Can you work these out from the model? Positions are in its coordinate system, mm. Face numbers are marked on the shaded views. A direction names the side the tool comes from. Give positions to 0.01 mm unless a question says otherwise; leave off trailing zeros. Write each loop counter-clockwise with the first axis right and the second up, starting at its lowest first coordinate (ties: lowest second). Pieces come first, ordered by that corner, then holes. Notation, with made-up numbers: (61, -31.75) - (119, -31.75) arc R18 cw to (119, -13.75) - close; hole circle Ø11 at (50, 65.5). An arc over 180 degrees is marked (long way). Use a Markdown table: item, result. Add a question column.
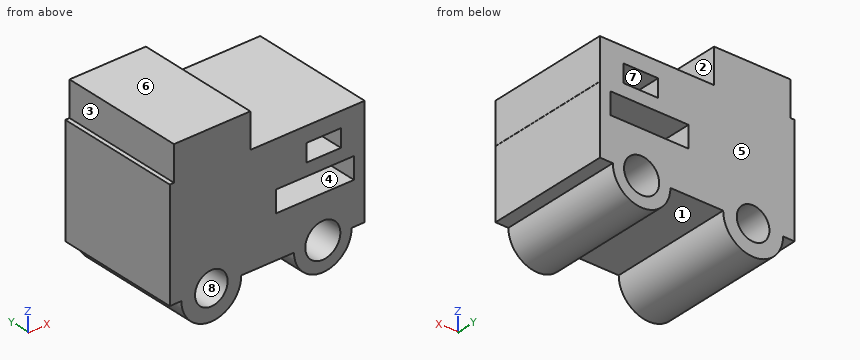
```python
from build123d import *

# Parameters (mm, degrees)
F0_W     = 21.6928645968
F0_H     = 12.4372411519
F0_W_2   = 24.2960043252
F0_W_3   = 53.6649217829
F0_H_2   = 15.3809413314
F0_W_4   = 54.884574376
F0_H_3   = 15.0760281831
F1_DEPTH = 25.4
F2_DEPTH = 62.738
F3_DEPTH = 71.374


with BuildPart() as f1:
    # F0 (on Front) → F1 (new body)
    with BuildSketch(Plane.XZ):
        Polygon((-61.0292442143, 47.0119267702), (-61.0292442143, 18.3321516961), (75.8868977427, 18.3321516961), (75.9811550379, 18.3321516961), (75.9811550379, 47.0119267702), align=None)
        with Locations((-32.8727662563, 29.9694752321)):
            Rectangle(F0_W, F0_H, mode=Mode.SUBTRACT)
        with Locations((47.1015777439, 29.9694752321)):
            Rectangle(F0_W_2, F0_H, mode=Mode.SUBTRACT)
        with BuildLine():
            Line((75.8868977427, 18.3321516961), (-61.0292442143, 18.3321516961))
            Line((-61.0292442143, 18.3321516961), (-61.0292442143, -29.6469051391))
            Line((-61.0292442143, -29.6469051391), (-52.8746465882, -29.6469051391))
            ThreePointArc((-52.8746465882, -29.6469051391), (-31.816188246, -8.5884467969), (-10.7577299038, -29.6469051391))
            Line((-10.7577299038, -29.6469051391), (26.3103456442, -29.6469051391))
            ThreePointArc((26.3103456442, -29.6469051391), (46.5673431754, -9.3899076079), (66.8243407066, -29.6469051391))
            Line((66.8243407066, -29.6469051391), (75.8868977427, -29.6469051391))
            Line((75.8868977427, -29.6469051391), (75.8868977427, 18.3321516961))
        make_face()
        with Locations((-31.2481601723, 7.6904706657)):
            Rectangle(F0_W_3, F0_H_2, mode=Mode.SUBTRACT)
        with Locations((41.0165307112, 7.5380140916)):
            Rectangle(F0_W_4, F0_H_3, mode=Mode.SUBTRACT)
        with BuildLine():
            ThreePointArc((-10.7577299038, -29.6469051391), (-31.816188246, -8.5884467969), (-52.8746465882, -29.6469051391))
            Line((-52.8746465882, -29.6469051391), (-43.2868667506, -29.6469051391))
            ThreePointArc((-43.2868667506, -29.6469051391), (-31.816188246, -18.1762266345), (-20.3455097415, -29.6469051391))
            Line((-20.3455097415, -29.6469051391), (-10.7577299038, -29.6469051391))
        make_face()
        with BuildLine():
            Line((-43.2868667506, -29.6469051391), (-52.8746465882, -29.6469051391))
            ThreePointArc((-52.8746465882, -29.6469051391), (-31.816188246, -50.7053634813), (-10.7577299038, -29.6469051391))
            Line((-10.7577299038, -29.6469051391), (-20.3455097415, -29.6469051391))
            ThreePointArc((-20.3455097415, -29.6469051391), (-31.816188246, -41.1175836436), (-43.2868667506, -29.6469051391))
        make_face()
        with BuildLine():
            ThreePointArc((26.3103456442, -29.6469051391), (46.5673431754, -49.9039026703), (66.8243407066, -29.6469051391))
            Line((66.8243407066, -29.6469051391), (58.8957230989, -29.6469051391))
            ThreePointArc((58.8957230989, -29.6469051391), (46.5673431754, -41.9752850626), (34.2389632519, -29.6469051391))
            Line((34.2389632519, -29.6469051391), (26.3103456442, -29.6469051391))
        make_face()
        with BuildLine():
            Line((58.8957230989, -29.6469051391), (66.8243407066, -29.6469051391))
            ThreePointArc((66.8243407066, -29.6469051391), (46.5673431754, -9.3899076079), (26.3103456442, -29.6469051391))
            Line((26.3103456442, -29.6469051391), (34.2389632519, -29.6469051391))
            ThreePointArc((34.2389632519, -29.6469051391), (46.5673431754, -17.3185252156), (58.8957230989, -29.6469051391))
        make_face()
    extrude(amount=F1_DEPTH)

    # F2 (add): a face of the model
    f2_faces = [f1.faces().sort_by_distance(p)[0] for p in [
        (7.2714959642, 0, 4.1694288848),
    ]]
    extrude(f2_faces, amount=F2_DEPTH)

    # F3 (add): faces of the model
    f3_faces = [f1.faces().sort_by_distance(p)[0] for p in [
        (-31.2481601723, -12.7, 0),
        (-31.2481601723, 31.369, 0),
    ]]
    extrude(f3_faces, amount=F3_DEPTH)


solid = f1.part
```
Q1. Suppose I cut it at D-D (x = 42). Please give me the cut outline in (y, z), and give its area (3 significant figures).
Q2. On a 3-axis mill with a long thin cutter (end or side, diameter ignored), from which of +Z, -Z, +X, -X, +Y, -Y can I reach the whole of each face in a straight line? I mean the marked faces 1, 2, 3 and 4. Say none if no direction works.
Q3. Suppose I cut it at A-A (y = -10.5). Please give me the cut outline in (x, z).
Q4. Suppose I cut it at C-C (x = 16). Please give me the cut outline in (y, z), and give its area (3 significant figures).
Q5. I'm going to push flat-ended pins straight in: P1, Ø7.5, axis at x = 50.5, y = 0, coming from the +Z side; P2, Ø2, axis at x = 47, y = 1.5, coming from the -Z side; P3, Ø2, axis at x = 34.5, z = 15, coming from the +Y side; P4, Ø8, axis at x = -34.5, y = 5.5, coming from the -Z side. Where does each tip first touch, or does it pass through?
Q6. Suppose I cut it at B-B (z = 27). Please give me the cut outline in (x, y).
Q7. If we mould it in two halves opening along Z, with no side actions, what happens to the marked faces 5, 6, 7 and 8? For each: released by +Z, released by -Z, zero draft, split by the parting line, or undercut.
Q8. If I drill on probe 1 along Z at (x, y) = (20, 6); probe 2 along X at (y, z) = (57.5, -33.5); probe 3 along X at (y, z) = (30, 14.5), over which ranges is the centre line in solid material (lowest first)? Write a range as [from, to].
Derived:
| question | item | result |
|---|---|---|
| 1 | outline | (-25.4, -49.38) - (62.74, -49.38) - (62.74, -41.1) - (-25.4, -41.1) - close; (-25.4, -18.2) - (62.74, -18.2) - (62.74, 0) - (-25.4, 0) - close; (-25.4, 15.08) - (62.74, 15.08) - (62.74, 23.75) - (-25.4, 23.75) - close; (-25.4, 36.19) - (62.74, 36.19) - (62.74, 47.01) - (-25.4, 47.01) - close |
| 1 | area | 4,050 mm² |
| 2 | face 1 | -Z, +Y, -Y |
| 2 | face 2 | +Z, +X, +Y, -Y |
| 2 | face 3 | +Z, -X, +Y, -Y |
| 2 | face 4 | +Y, -Y |
| 3 | outline | (-61.03, -29.65) - (-52.87, -29.65) arc R21.06 ccw to (-10.76, -29.65) - (26.31, -29.65) arc R20.26 ccw to (66.82, -29.65) - (75.89, -29.65) - (75.89, 18.33) - (75.98, 18.33) - (75.98, 47.01) - (-4.42, 47.01) - (-4.42, 71.37) - (-58.08, 71.37) - (-58.08, 47.01) - (-61.03, 47.01) - close; hole circle Ø22.94 at (-31.82, -29.65); hole (13.57, 0) - (68.46, 0) - (68.46, 15.08) - (13.57, 15.08) - close; hole circle Ø24.66 at (46.57, -29.65); hole (34.95, 23.75) - (59.25, 23.75) - (59.25, 36.19) - (34.95, 36.19) - close |
| 4 | outline | (-25.4, -29.65) - (62.74, -29.65) - (62.74, 0) - (-25.4, 0) - close; (-25.4, 15.08) - (62.74, 15.08) - (62.74, 47.01) - (-25.4, 47.01) - close |
| 4 | area | 5,430 mm² |
| 5 | P1 | z = 47.01 |
| 5 | P2 | z = -49.9 |
| 5 | P3 | y = 62.74 |
| 5 | P4 | z = -50.71 |
| 6 | outline | (-61.03, -25.4) - (34.95, -25.4) - (34.95, 62.74) - (-61.03, 62.74) - close; (59.25, -25.4) - (75.98, -25.4) - (75.98, 62.74) - (59.25, 62.74) - close |
| 7 | face 5 | zero draft |
| 7 | face 6 | released by +Z |
| 7 | face 7 | undercut |
| 7 | face 8 | undercut |
| 8 | probe 1 | [-29.65, 0], [15.08, 47.01] |
| 8 | probe 2 | [-52.52, -42.62], [-21.01, -11.11], [26.68, 34.86], [58.28, 66.45] |
| 8 | probe 3 | [-61.03, 13.57], [68.46, 75.89] |
